```python
from build123d import *

# Parameters (mm, degrees)
SKETCH030_R         = 11.1
SKETCH030_R_2       = 1.65
PAD018_DEPTH        = 6
PAD021_DEPTH        = 10
SKETCH032_R         = 5
POCKET013_DEPTH     = 2
HOLE004_D           = 3.4
HOLE004_CSINK_D     = 6.1
HOLE004_CSINK_ANGLE = 90


with BuildPart() as part:
    # Sketch030 → Pad018 (new body)
    with BuildSketch(Plane.XY):
        with BuildLine():
            Line((-30, -10), (-30, 10))
            Line((-30, 10), (-30, 38))
            Line((-30, 38), (-8.506442, 48.100841))
            ThreePointArc((20, 30), (10.720801, 46.883851), (-8.506442, 48.100841))
            Line((20, 30), (20, 0))
            ThreePointArc((10, -10), (17.071068, -7.071068), (20, 0))
            Line((10, -10), (-30, -10))
        make_face()
        with Locations((0, 30)):
            Circle(SKETCH030_R, mode=Mode.SUBTRACT)
        with Locations((-9.899495, 39.899495)):
            Circle(SKETCH030_R_2, mode=Mode.SUBTRACT)
        with Locations((9.899495, 39.899495)):
            Circle(SKETCH030_R_2, mode=Mode.SUBTRACT)
        with Locations((9.899495, 20.100505)):
            Circle(SKETCH030_R_2, mode=Mode.SUBTRACT)
        with Locations((-9.899495, 20.100505)):
            Circle(SKETCH030_R_2, mode=Mode.SUBTRACT)
        with BuildLine():
            ThreePointArc((-25, 2.25), (-27.25, 0), (-25, -2.25))
            Line((-25, -2.25), (-10, -2.25))
            ThreePointArc((-10, -2.25), (-7.75, 0), (-10, 2.25))
            Line((-25, 2.25), (-10, 2.25))
        make_face(mode=Mode.SUBTRACT)
        with BuildLine():
            ThreePointArc((0, 2.25), (-2.25, 0), (0, -2.25))
            Line((0, -2.25), (15, -2.25))
            ThreePointArc((15, -2.25), (17.25, 0), (15, 2.25))
            Line((0, 2.25), (15, 2.25))
        make_face(mode=Mode.SUBTRACT)
    extrude(amount=PAD018_DEPTH)

    # Sketch036 → Pad021 (join)
    with BuildSketch(Plane.XY):
        with BuildLine():
            Line((20, 10), (20, 0))
            ThreePointArc((10, -10), (17.071068, -7.071068), (20, 0))
            Line((10, -10), (-30, -10))
            Line((-30, -10), (-30, 10))
            Line((-30, 38), (-30, 10))
            Line((-20, 38), (-30, 38))
            Line((-20, 10), (-20, 38))
            Line((-20, 10), (20, 10))
        make_face()
        with BuildLine():
            ThreePointArc((-25, 2.25), (-27.25, 0), (-25, -2.25))
            Line((-25, -2.25), (-10, -2.25))
            ThreePointArc((-10, -2.25), (-7.75, 0), (-10, 2.25))
            Line((-25, 2.25), (-10, 2.25))
        make_face(mode=Mode.SUBTRACT)
        with BuildLine():
            ThreePointArc((0, 2.25), (-2.25, 0), (0, -2.25))
            Line((0, -2.25), (15, -2.25))
            ThreePointArc((15, -2.25), (17.25, 0), (15, 2.25))
            Line((0, 2.25), (15, 2.25))
        make_face(mode=Mode.SUBTRACT)
    extrude(amount=-PAD021_DEPTH)

    # Sketch032 → Pocket013 (cut)
    with BuildSketch(Plane.YZ.offset(-30)):
        with Locations((0, -3)):
            Circle(SKETCH032_R)
        with Locations((30, -3)):
            Circle(SKETCH032_R)
    extrude(amount=POCKET013_DEPTH, mode=Mode.SUBTRACT)

    # Hole004 (through all)
    with Locations(Plane.XY.offset(6)):
        with Locations((9.899495, 39.899495), (-9.899495, 39.899495), (-9.899495, 20.100505), (9.899495, 20.100505)):
            CounterSinkHole(HOLE004_D / 2, HOLE004_CSINK_D / 2, counter_sink_angle=HOLE004_CSINK_ANGLE)


solid = part.part
```
Geometry check sheet. Reference: the model listing, model coordinates, mm. A direction names the side the tool comes from. Give positions to 0.01 mm unless a question says otherwise; leave off trailing zeros. Write each loop counter-clockwise with the first axis right and the second up, starting at its lowest first coordinate (ties: lowest second). Pieces come first, ordered by that corner, then holes. Notation, with made-up numbers: (65.5, 84.5) -> (86.5, 84.5) arc R16 ccw to (86.5, 100.5) -> close; hole circle Ø9 at (61, 73). An arc over 180 degrees is marked (long way). Use one line per item in the form item = value.
Item 1: Depth check by flat-ended pin: pin 1 Ø3 at (y, z) = (31.5, -2) entering from -X; pin 2 Ø5 at (x, z) = (-26.5, -4.5) entering from +Y; pin 3 Ø4.5 at (x, z) = (-15, -3) entering from +Y. Enter the tip coordinate at first touch or a pass-through.
Results list:
pin_1 = -28
pin_2 = 38
pin_3 = 10
Item 2: Sectioned sample at C-C on y = -1.5. Enter the section's corners in (x, z).
Results list:
outline = (-30, -10) -> (-26.68, -10) -> (-26.68, 6) -> (-30, 6) -> (-30, 1.77) -> (-28, 1.77) -> (-28, -7.77) -> (-30, -7.77) -> close; (-8.32, -10) -> (-1.68, -10) -> (-1.68, 6) -> (-8.32, 6) -> close; (16.68, -10) -> (19.89, -10) -> (19.89, 6) -> (16.68, 6) -> close
Item 3: Mould release check, pull along Y, two halves, no side actions. Record for faces 1 (the cylindrical face through (10.96, 46.73, 2.96)), 2 (the flat face through (-5, 14, 6)), 3 (the cylindrical face through (-27.25, 0.05, -1.89)): released by +Y, released by -Y, zero draft, split by the parting line, or undercut.
Results list:
face_1 = released by +Y
face_2 = zero draft
face_3 = undercut
Item 4: Access from +Z, -Z, +X, -X, +Y, -Y to the whole of each face (thin tool, end or side, straight path). Record for faces 4 (the cylindrical face through (16.99, -7.15, -1.89)), 5 (the flat face through (0, 10, -5)), 6 (the cylindrical face through (17.25, -0.05, -1.89)), 7 (the flat face through (20, 12, 2)), 8 (the flat face through (-28, 0, -3)).
Results list:
face_4 = +Z, -Z, +X, -Y
face_5 = -Z, +X, +Y
face_6 = +Z, -Z
face_7 = +Z, -Z, +X, +Y, -Y
face_8 = -X
Item 5: Scan lines: line 1 (Z direction, x = -28.75, y = 0); line 2 (Y direction, x = 1.5, z = 5.25); line 3 (Y direction, x = 2, z = 0.5). Record each from-to range of solid material in increasing order.
Results list:
line_1 = -10 to -8, 2 to 6
line_2 = -10 to -2.25, 2.25 to 19, 41 to 49.94
line_3 = -10 to -2.25, 2.25 to 19.08, 40.92 to 49.9
Item 6: Sectioned sample at A-A on z = -9. Enter the section's corners in (x, y).
Results list:
outline = (-30, -10) -> (10, -10) arc R10 ccw to (20, 0) -> (20, 10) -> (-20, 10) -> (-20, 38) -> (-30, 38) -> close; hole (-25, -2.25) -> (-10, -2.25) arc R2.25 ccw to (-10, 2.25) -> (-25, 2.25) arc R2.25 ccw to start; hole (0, -2.25) -> (15, -2.25) arc R2.25 ccw to (15, 2.25) -> (0, 2.25) arc R2.25 ccw to start
Item 7: Sectioned sample at D-D on y = 33. Enter the section's corners in (x, z).
Results list:
outline = (-30, -10) -> (-20, -10) -> (-20, 0) -> (-10.69, 0) -> (-10.69, 6) -> (-30, 6) -> (-30, 1) -> (-28, 1) -> (-28, -7) -> (-30, -7) -> close; (10.69, 0) -> (19.77, 0) -> (19.77, 6) -> (10.69, 6) -> close
Item 8: Sectioned sample at B-B on x = -26. Enter the section's corners in (y, z), plus the area to 3 significant figures.
Results list:
outline = (-10, -10) -> (-2.02, -10) -> (-2.02, 6) -> (-10, 6) -> close; (2.02, -10) -> (38, -10) -> (38, 0) -> (39.88, 0) -> (39.88, 6) -> (2.02, 6) -> close
area = 715 mm2
